Autodesk Inventor part; units mm, degrees
ref_plane "YZ Plane" through (0, 0, 0) normal (1, 0, 0) x (0, 1, 0)
ref_plane "XZ Plane" through (0, 0, 0) normal (0, 1, 0) x (-1, 0, 0)
ref_plane "XY Plane" through (0, 0, 0) normal (0, 0, 1) x (1, 0, 0)
sketch "Sketch1" plane through (0, 0, 0) normal (0, 1, 0) x (-1, 0, 0)
  line L0 (-231.775, 282.575) -> (231.775, 282.575)
  line L1 (231.775, 282.575) -> (231.775, -282.575)
  line L2 (231.775, -282.575) -> (-231.775, -282.575)
  line L3 (-231.775, -282.575) -> (-231.775, 282.575)
  line L4 (-231.775, 282.575) -> (231.775, -282.575) construction
  line L5 (231.775, 282.575) -> (-231.775, -282.575) construction
  point P0 (0, 0)
  dimension "d0" = 565.15
  dimension "d1" = 463.55
extrude "Extrusion1" add sketch "Sketch1" along normal blind 158.75 and the other way blind 6.35
sketch "Sketch2" plane through (0, 158.75, 0) normal (0, 1, 0) x (1, 0, 0)
  line L0 (228.6, -277.8125) -> (-228.6, -277.8125)
  line L1 (-228.6, -277.8125) -> (-228.6, 277.8125)
  line L2 (-228.6, 277.8125) -> (228.6, 277.8125)
  line L3 (228.6, 277.8125) -> (228.6, -277.8125)
  line L4 (228.6, -277.8125) -> (-228.6, 277.8125) construction
  line L5 (-228.6, -277.8125) -> (228.6, 277.8125) construction
  point P0 (0, 0)
  dimension "d4" = 555.625
  dimension "d5" = 457.2
extrude "Extrusion2" cut sketch "Sketch2" against normal blind 158.75
properties part number "Pelican box"
Could you check a few things on this model? Use its own coordinates, in mm. A direction names the side the tool comes from. Round coordinates to 2 decimals unless told otherwise and drop trailing zeros. Loops run counter-clockwise (first coordinate to the right, second up) from the corner with the lowest first, then second, coordinate; pieces in that order, holes last. Notation, with made-up numbers: (41, 46.25) -> (69, 46.25) arc R9 ccw to (69, 54.25) -> close; hole circle Ø9 at (-5, -25). An arc over 180 degrees is marked (long way). Put each result on its own line as item: value.
Q1. Which directions (+Z, -Z, +X, -X, +Y, -Y) give clear straight access to the entire face, cutting with the end or side of a thin tool? Please do faces 5 (the flat face through (-3, 80, -277.812)), 6 (the flat face through (3, -6.35, 4)).
Checks:
face 5: +Y
face 6: +Z, -Z, +X, -X, -Y
Q2. I want a section at B-B on z = 136.5. Write out the boundary of the cut face in (x, y) (3 decimals), and give its area (3 significant figures).
Checks:
outline: (-231.775, -6.35) -> (231.775, -6.35) -> (231.775, 158.75) -> (228.6, 158.75) -> (228.6, 0) -> (-228.6, 0) -> (-228.6, 158.75) -> (-231.775, 158.75) -> close
area: 3,950 mm2
Q3. Please list where these lines run through material, in increasing order: line 1 (X direction, y = 60.5, z = -138) (3 decimals); line 2 (Z direction, x = 6, y = 131.5) (1 decimal); line 3 (Y direction, x = 146, z = 22.5). Write a range as from..to.
Checks:
line 1: -231.775..-228.6, 228.6..231.775
line 2: -282.6..-277.8, 277.8..282.6
line 3: -6.35..0
Q4. Thinking about a two-plate mould opening in Z: for faces 1 (the flat face through (-3, 0, -4)), 2 (the flat face through (-3, 75, -282.575)), 3 (the flat face through (228.6, 80, -4)), 4 (the flat face through (3, 75, 282.575)), which applies, pulls with the +Z half, pulls with the -Z half, needs draft (parallel to the pull), parting line crosses it, or undercut?
Checks:
face 1: undercut
face 2: pulls with the -Z half
face 3: undercut
face 4: pulls with the +Z half
Q5. I want a section at A-A on y = 86. Write out the boundary of the cut face in (x, z) (1 decimal).
Checks:
outline: (-231.8, -282.6) -> (231.8, -282.6) -> (231.8, 282.6) -> (-231.8, 282.6) -> close; hole (-228.6, -277.8) -> (228.6, -277.8) -> (228.6, 277.8) -> (-228.6, 277.8) -> close
